Autodesk Inventor part; units mm, degrees
ref_plane "YZ Plane" through (0, 0, 0) normal (1, 0, 0) x (0, 1, 0)
ref_plane "XZ Plane" through (0, 0, 0) normal (0, 1, 0) x (-1, 0, 0)
ref_plane "XY Plane" through (0, 0, 0) normal (0, 0, 1) x (1, 0, 0)
sketch "Sketch1" plane through (0, 0, 0) normal (1, 0, 0) x (0, 1, 0)
  circle A0 centre (0, 0) radius 4
  arc A1 (6.1319, -1.65) -> (6.1319, 1.65) centre (0, 0) ccw
  line L0 (0, 4) -> (3.0659, 4)
  line L1 (0, -4) -> (3.0659, -4)
  arc A2 (6.1319, 1.65) -> (3.0659, 4) centre (3.0659, 0.825) ccw
  arc A3 (3.0659, -4) -> (6.1319, -1.65) centre (3.0659, -0.825) ccw
  point P0 (4.9318, 4)
  point P1 (4.9318, -4)
  dimension "d0" = 8
  dimension "d1" = 12.7
  dimension "d2" = 3.175
extrude "Extrusion1" add sketch "Sketch1" along normal mid plane 88.2904 contours A0
extrude "Extrusion2" add sketch "Sketch1" along normal mid plane 50.8 contours A0 L0 A2 A1 A3 L1
sketch "Sketch2" plane through (44.1452, 0, 0) normal (1, 0, 0) x (0, 0, -1)
  circle A0 centre (0, 0) radius 4
  line L0 (0, 0) -> (0, 3.3434)
  line L1 (0, 3.3434) -> (0.7706, 3.3434)
  line L2 (0.7706, 3.3434) -> (0.7706, 3.9251)
  line L3 (0, 3.3434) -> (-0.7706, 3.3434)
  line L4 (-0.7706, 3.3434) -> (-0.7706, 3.9251)
extrude "Extrusion3" cut sketch "Sketch2" against normal blind 6.35 contours L2 L1 L3 L4 A0 picked at (0.343, 3.5595)
properties part number "Cam Shaft Test"
For this review, take the finished solid that the model builds, in its own axes (mm). A direction names the side the tool comes from. Coordinates: 2 decimals unless noted, no trailing zeros. Write each loop counter-clockwise with the first axis right and the second up, starting at its lowest first coordinate (ties: lowest second). Pieces come first, ordered by that corner, then holes. Notation, with made-up numbers: (4, 36) - (54, 36) arc R27 cw to (54, 64) - close; hole circle Ø5 at (61, 31). An arc over 180 degrees is marked (long way). Answer in a Markdown table with one row per item. Add a question column.
Q1. We need section C-C, the plane x = 16. State the section outline as (y, z) points, and give its area (3 significant figures).
Q2. We need section D-D, the plane y = -1.75. State the section outline as (x, z) points, and give its area (3 significant figures).
Q3. For P1, Ø1.5, axis at x = -32, z = -1.5, coming from the +Y side; P2, Ø0.5, axis at x = 39.5, y = 3.5, coming from the -Z side; P3, Ø1.2, axis at x = 40, z = 0, coming from the +Y side, all flat-tipped, find the tip position at first contact; note any pin that passes through.
Q4. For probe 1 along X at (y, z) = (6, -0.75); probe 2 along Y at (x, z) = (28.5, 0); probe 3 along Y at (x, z) = (-33, -2), list the stretches that pass through material, from the lowest coordinate up.
Q5. We need section A-A, the plane z = 0. State the section outline as (x, y) points.
Q6. We need section B-B, the plane x = 35. State the section outline as (y, z) points.
Q7. Tool access review of faces 1 (the flat face through (-25.4, 5, 0)), 2 (the flat face through (25.4, 5, 0)), 3 (the cylindrical face through (-1, -4, 0)), 4 (the flat face through (-44.145, 0, 0)): name each direction out of +Z, -Z, +X, -X, +Y, -Y from which nothing blocks a thin tool from reaching the whole face with its end or side.
Answer list:
| question | item | result |
|---|---|---|
| 1 | outline | (0, -4) - (3.07, -4) arc R3.18 ccw to (6.13, -1.65) arc R6.35 ccw to (6.13, 1.65) arc R3.17 ccw to (3.07, 4) - (0, 4) arc R4 ccw to start |
| 1 | area | 70.9 mm2 |
| 2 | outline | (-44.15, -3.6) - (44.15, -3.6) - (44.15, 3.6) - (-44.15, 3.6) - close |
| 2 | area | 635 mm2 |
| 3 | P1 | stops at y = 3.93 |
| 3 | P2 | stops at z = -2.33 |
| 3 | P3 | stops at y = 3.34 |
| 4 | probe 1 | x = -25.4 to 25.4 |
| 4 | probe 2 | y = -4 to 4 |
| 4 | probe 3 | y = -3.46 to 3.46 |
| 5 | outline | (-44.15, -4) - (44.15, -4) - (44.15, 3.34) - (37.8, 3.34) - (37.8, 4) - (25.4, 4) - (25.4, 6.35) - (-25.4, 6.35) - (-25.4, 4) - (-44.15, 4) - close |
| 6 | outline | circle Ø8 at (0, 0) |
| 7 | face 1 | -X, +Y |
| 7 | face 2 | +X, +Y |
| 7 | face 3 | none |
| 7 | face 4 | +Z, -Z, -X, +Y, -Y |
